Read the model definition and answer for the solid it produces. Units are mm, in the model's axes. Face numbers are marked on the shaded views. A direction names the side the tool comes from. Give positions to 0.01 mm unless a question says otherwise; leave off trailing zeros. Order: outer loops, then holes, each group sorted by start corner. A loop starts at its lowest first (then second) coordinate and runs counter-clockwise, first axis right, second up.
```python
from build123d import *

# Parameters (mm, degrees)
SKETCH1_R           = 1.3
BOSS_EXTRUDE1_DEPTH = 2.5
SKETCH2_R           = 1.3
BOSS_EXTRUDE2_DEPTH = 4
SKETCH3_R           = 1.3
BOSS_EXTRUDE3_DEPTH = 2.25
CUT_EXTRUDE1_DEPTH  = 5
CUT_EXTRUDE2_DEPTH  = 3.25
BOSS_EXTRUDE4_DEPTH = 8
CUT_EXTRUDE3_REACH  = 55.54
CUT_EXTRUDE4_DEPTH  = 4.6
CHAMFER1_SIZE       = 1
SKETCH10_W          = 2.8
SKETCH10_H          = 2.8
CUT_EXTRUDE6_DEPTH  = 1.95
SKETCH12_W          = 1.175
SKETCH12_H          = 3
CUT_EXTRUDE7_DEPTH  = 2.5
BOSS_EXTRUDE6_START = 1.175
BOSS_EXTRUDE6_DEPTH = 1.175


with BuildPart() as part:
    # Sketch1 → Boss-Extrude1 (new body)
    with BuildSketch(Plane.XY):
        Polygon((-5, 25.75), (5, 25.75), (7.75, 20.25), (7.75, 0.25), (10.2, 0.25), (10.2, -25.75), (-10.2, -25.75), (-10.2, 0.25), (-7.75, 0.25), (-7.75, 20.25), align=None)
        with Locations((0, 22.9)):
            Circle(SKETCH1_R, mode=Mode.SUBTRACT)
        with Locations((0.9, -18.85)):
            Circle(SKETCH1_R, mode=Mode.SUBTRACT)
    extrude(amount=BOSS_EXTRUDE1_DEPTH)

    # Sketch2 → Boss-Extrude2 (add)
    with BuildSketch(Plane.XY.offset(2.5)):
        Polygon((-7.75, 3.25), (7.75, 3.25), (7.75, 20.25), (5, 25.75), (-5, 25.75), (-7.75, 20.25), align=None)
        with Locations((0, 22.9)):
            Circle(SKETCH2_R, mode=Mode.SUBTRACT)
    extrude(amount=BOSS_EXTRUDE2_DEPTH)

    # Sketch3 → Boss-Extrude3 (add)
    with BuildSketch(Plane.XY.offset(2.5)):
        Polygon((-1.1, -15.35), (2.9, -15.35), (4.4, -16.85), (4.4, -22.35), (-2.6, -22.35), (-2.6, -16.85), align=None)
        with Locations((0.9, -18.85)):
            Circle(SKETCH3_R, mode=Mode.SUBTRACT)
    extrude(amount=BOSS_EXTRUDE3_DEPTH)

    # Sketch4 → Cut-Extrude1 (cut)
    with BuildSketch(Plane(origin=(0, 0, 0), x_dir=(-1, 0, 0), z_dir=(0, 0, -1))):
        Polygon((2.915618859, 22.9), (1.45780943, 25.425), (-1.45780943, 25.425), (-2.915618859, 22.9), (-1.45780943, 20.375), (1.45780943, 20.375), align=None)
    extrude(amount=-CUT_EXTRUDE1_DEPTH, mode=Mode.SUBTRACT)

    # Sketch5 → Cut-Extrude2 (cut)
    with BuildSketch(Plane(origin=(0, 0, 0), x_dir=(-1, 0, 0), z_dir=(0, 0, -1))):
        Polygon((2.015618859, -18.85), (0.55780943, -16.325), (-2.35780943, -16.325), (-3.815618859, -18.85), (-2.35780943, -21.375), (0.55780943, -21.375), align=None)
    extrude(amount=-CUT_EXTRUDE2_DEPTH, mode=Mode.SUBTRACT)

    # Sketch6 → Boss-Extrude4 (add)
    with BuildSketch(Plane.XY.offset(2.5)):
        Polygon((-7.75, 0.25), (-10.2, 0.25), (-10.2, -25.75), (10.2, -25.75), (10.2, 0.25), (7.75, 0.25), (7.75, -23.3), (-7.75, -23.3), align=None)
    extrude(amount=BOSS_EXTRUDE4_DEPTH)

    # Sketch8 → Cut-Extrude3 (cut, up to next)
    with BuildSketch(Plane.XZ.offset(25.75), mode=Mode.PRIVATE) as cut_extrude3_sk1:
        with BuildLine():
            Line((-7.75, 10.5), (-7.75, 7.25))
            ThreePointArc((-7.75, 7.25), (-7.530330086, 6.719669914), (-7, 6.5))
            Line((-7, 6.5), (-5.5, 6.5))
            ThreePointArc((-5.5, 6.5), (-4.969669914, 6.719669914), (-4.75, 7.25))
            Line((-4.75, 7.25), (-4.75, 10.5))
            Line((-4.75, 10.5), (-7.75, 10.5))
        make_face()
    cut_extrude3_tool1 = extrude(cut_extrude3_sk1.sketch, amount=-CUT_EXTRUDE3_REACH, mode=Mode.PRIVATE) & part.part
    # Sketch8 → Cut-Extrude3 (cut, up to next)
    with BuildSketch(Plane.XZ.offset(25.75), mode=Mode.PRIVATE) as cut_extrude3_sk2:
        with BuildLine():
            Line((6.25, 10.5), (6.25, 7.25))
            ThreePointArc((6.25, 7.25), (7, 6.5), (7.75, 7.25))
            Line((7.75, 7.25), (7.75, 10.5))
            Line((7.75, 10.5), (6.25, 10.5))
        make_face()
    cut_extrude3_tool2 = extrude(cut_extrude3_sk2.sketch, amount=-CUT_EXTRUDE3_REACH, mode=Mode.PRIVATE) & part.part
    add(cut_extrude3_tool1.solids().sort_by_distance((-6.25, -25.75, 8.537624))[0], mode=Mode.SUBTRACT)
    add(cut_extrude3_tool2.solids().sort_by_distance((7, -25.75, 8.576826))[0], mode=Mode.SUBTRACT)

    # Sketch9 → Cut-Extrude4 (cut)
    with BuildSketch(Plane.XY.offset(10.5)):
        Polygon((-9.025, 0.25), (-10.2, 0.25), (-10.2, -25.75), (10.2, -25.75), (10.2, 0.25), (9.025, 0.25), (9.025, -24.575), (-9.025, -24.575), align=None)
    extrude(amount=-CUT_EXTRUDE4_DEPTH, mode=Mode.SUBTRACT)

    # Chamfer1
    chamfer1_edges = [part.edges().sort_by_distance(p)[0] for p in [
        (-7.75, 0.25, 1.25),
        (7.75, 0.25, 1.25),
        (-10.2, -25.75, 2.95),
        (-10.2, 0.25, 2.95),
        (10.2, 0.25, 2.95),
        (10.2, -25.75, 2.95),
    ]]
    chamfer(chamfer1_edges, length=CHAMFER1_SIZE)

    # Sketch10 → Cut-Extrude6 (cut)
    with BuildSketch(Plane.ZY.offset(10.2)):
        with Locations((2.95, -6.75)):
            Rectangle(SKETCH10_W, SKETCH10_H)
        with Locations((2.95, -18.75)):
            Rectangle(SKETCH10_W, SKETCH10_H)
    extrude(amount=-CUT_EXTRUDE6_DEPTH, mode=Mode.SUBTRACT)

    # Sketch12 → Cut-Extrude7 (cut)
    with BuildSketch(Plane.XY.offset(5.9)):
        with Locations((-9.6125, -3.25)):
            Rectangle(SKETCH12_W, SKETCH12_H)
        with Locations((9.6125, -3.25)):
            Rectangle(SKETCH12_W, SKETCH12_H)
    extrude(amount=-CUT_EXTRUDE7_DEPTH, mode=Mode.SUBTRACT)

    # Sketch13 → Boss-Extrude6 (add)
    with BuildSketch(Plane.XZ.offset(24.575).offset(BOSS_EXTRUDE6_START)):
        with BuildLine():
            Line((-7.65, 6.875834261), (-7.65, 5.9))
            Line((-7.65, 5.9), (-4.85, 5.9))
            Line((-4.85, 5.9), (-4.85, 6.875834261))
            ThreePointArc((-4.85, 6.875834261), (-5.124583101, 6.600721822), (-5.5, 6.5))
            Line((-5.5, 6.5), (-7, 6.5))
            ThreePointArc((-7, 6.5), (-7.375416899, 6.600721822), (-7.65, 6.875834261))
        make_face()
        with BuildLine():
            Line((6.35, 6.875834261), (6.35, 5.9))
            Line((6.35, 5.9), (7.65, 5.9))
            Line((7.65, 5.9), (7.65, 6.875834261))
            ThreePointArc((7.65, 6.875834261), (7, 6.5), (6.35, 6.875834261))
        make_face()
    extrude(amount=-BOSS_EXTRUDE6_DEPTH)


solid = part.part
```
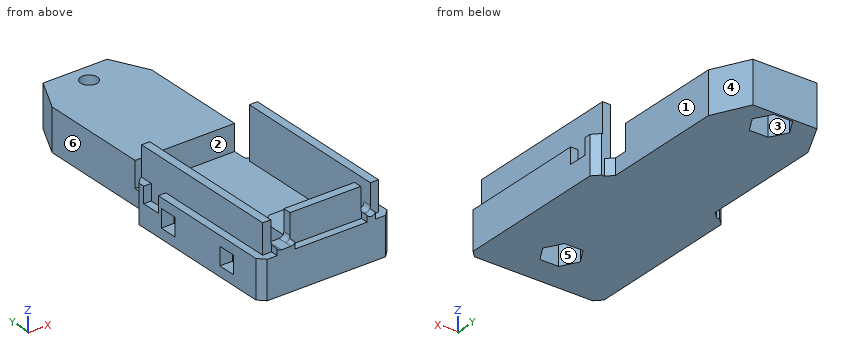
1) Consider L1, parallel to X at y = -18.85, z = 3.95; L2, parallel to Y at x = 0, z = 5.85; L3, parallel to Y at x = 0.9, z = 4.3 (3 decimals). Determine where each line is inside the solid, lowest interval first.
Final values:
L1: x = -8.25 to -7.75, -2.6 to -0.4, 2.2 to 4.4, 7.75 to 10.2
L2: y = -25.75 to -23.3, 3.25 to 21.6, 24.2 to 25.75
L3: y = -25.75 to -23.3, -22.35 to -20.15, -17.55 to -15.35, 3.25 to 20.375, 25.425 to 25.75
2) A tool of negligible diameter and unlimited length cuts with its end or side. For the marked faces 1, 2 and 3, from which of +Z, -Z, +X, -X, +Y, -Y can it reach the whole face along a straight path? Write none if from no direction.
Final values:
face 1: +Z, -Z, +X, +Y
face 2: +Z, +X, -X
face 3: -Z
3) The part is cut by section A-A on z = 8.75. Determine the outline of the cut face in (x, y) (3 decimals).
Final values:
outline: (-9.025, -24.575) - (-7.75, -24.575) - (-7.75, 0.25) - (-9.025, 0.25) - close; (-4.75, -24.575) - (6.25, -24.575) - (6.25, -23.3) - (-4.75, -23.3) - close; (7.75, -24.575) - (9.025, -24.575) - (9.025, 0.25) - (7.75, 0.25) - close
4) The part is cut by section D-D on x = -4. Determine the outline of the cut face in (y, z) (3 decimals).
Final values:
outline: (-25.75, 0) - (25.75, 0) - (25.75, 6.5) - (3.25, 6.5) - (3.25, 2.5) - (-23.3, 2.5) - (-23.3, 10.5) - (-24.575, 10.5) - (-24.575, 5.9) - (-25.75, 5.9) - close
5) The part is cut by section C-C on y = -3.5. Determine the outline of the cut face in (x, z) (3 decimals).
Final values:
outline: (-10.2, 0) - (10.2, 0) - (10.2, 3.4) - (9.025, 3.4) - (9.025, 10.5) - (7.75, 10.5) - (7.75, 2.5) - (-7.75, 2.5) - (-7.75, 10.5) - (-9.025, 10.5) - (-9.025, 3.4) - (-10.2, 3.4) - close
6) For a pull along Y with two mould halves and no side action, classify the marked faces 4, 5 and 6 as released by +Y, released by -Y, zero draft, split by the parting line, or undercut.
Final values:
face 4: released by +Y
face 5: undercut
face 6: zero draft
7) The part is cut by section B-B on x = 7. Determine the outline of the cut face in (y, z), and give its area (3 significant figures).
Final values:
outline: (-25.75, 0) - (21.75, 0) - (21.75, 6.5) - (3.25, 6.5) - (3.25, 2.5) - (-23.3, 2.5) - (-23.3, 6.5) - (-25.75, 6.5) - close
area: 203 mm2
8) Given pin 1 (1.3 mm diameter, centred on x = 9.5, y = -4, fed in from +Z); pin 2 (1.6 mm diameter, centred on x = -9, z = 2.5, fed in from +Y); pin 3 (2 mm diameter, centred on x = 7, y = 17, fed in from +Z); pin 4 (1 mm diameter, centred on y = 0, z = 8.5, fed in from +X) (3 decimals), each flat-ended and moving along its own axis, determine where each tip first touches the part or whether it passes through.
Final values:
pin 1: stops at z = 10.5
pin 2: stops at y = 0.8
pin 3: stops at z = 6.5
pin 4: stops at x = 9.025
